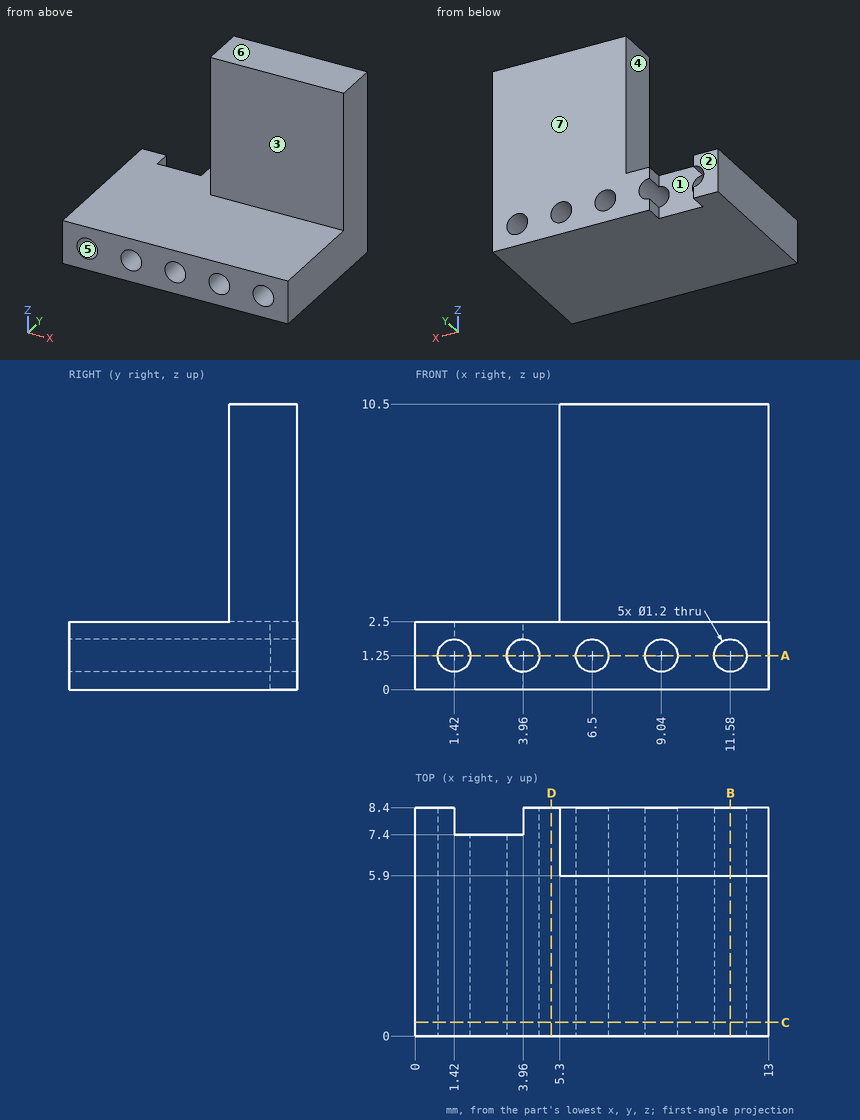
Input: dimensioned drawing with shaded views. Units: mm. Origin: part minimum x, y, z. A direction names the side the tool comes from. Give positions to 0.01 mm unless a question says otherwise; leave off trailing zeros. Loops run counter-clockwise (first coordinate to the right, second up) from the corner with the lowest first, then second, coordinate; pieces in that order, holes last. Notation, with made-up numbers: (6, 77) -> (62, 77) arc R18 ccw to (62, 91) -> close; hole circle Ø7 at (52.25, 7). An arc over 180 degrees is marked (long way). Use a Markdown table: item, result. Add a question column.
1) Section query B-B, the plane x = 11.58. Return the cut outline in (y, z), then the cut area to 3 significant figures.
2) Section query A-A, the plane z = 1.25. Return the cut outline in (x, y).
3) Reachability of the marked faces 1, 2, 3 and 4 from +Z, -Z, +X, -X, +Y, -Y: full face, straight path, thin tool, end or side. Return the list, or none.
4) First-contact query: pin 1 (0.8 mm diameter, centred on y = 7, z = 6, fed in from -X); pin 2 (3 mm diameter, centred on x = 6, z = 5.5, fed in from -Y); pin 3 (0.8 mm diameter, centred on x = 2.5, z = 1.5, fed in from +Y). Flat tips, straight axial feed; report the tip coordinate or a pass-through.
5) Section query C-C, the plane y = 0.5. Return the cut outline in (x, z).
6) Pull-direction query (Z, two-part tool) for the marked faces 5, 6 and 7; classes: +Z half, -Z half, draft (parallel to the pull), parting line (faces both ways), or undercut.
7) Line query: line 1 along X through (y, z) = (8.25, 1.25); line 2 along X through (y, z) = (4.75, 1.25); line 3 along Z through (x, y) = (4, 1.75). Output: solid intervals per line, ascending. Write a range as [from, to].
8) Section query D-D, the plane x = 5. Return the cut outline in (y, z).
Numbers:
| question | item | result |
|---|---|---|
| 1 | outline | (0, 0) -> (8.4, 0) -> (8.4, 0.65) -> (0, 0.65) -> close; (0, 1.85) -> (8.4, 1.85) -> (8.4, 10.5) -> (5.9, 10.5) -> (5.9, 2.5) -> (0, 2.5) -> close |
| 1 | area | 30.9 mm2 |
| 2 | outline | (0, 0) -> (0.82, 0) -> (0.82, 8.4) -> (0, 8.4) -> close; (2.02, 0) -> (3.36, 0) -> (3.36, 7.4) -> (2.02, 7.4) -> close; (4.56, 0) -> (5.9, 0) -> (5.9, 8.4) -> (4.56, 8.4) -> close; (7.1, 0) -> (8.44, 0) -> (8.44, 8.4) -> (7.1, 8.4) -> close; (9.64, 0) -> (10.98, 0) -> (10.98, 8.4) -> (9.64, 8.4) -> close; (12.18, 0) -> (13, 0) -> (13, 8.4) -> (12.18, 8.4) -> close |
| 3 | face 1 | +Z, -Z, +Y |
| 3 | face 2 | +Z, -Z, +X, -X, +Y |
| 3 | face 3 | +Z, +X, -X, -Y |
| 3 | face 4 | +Z, -X, +Y, -Y |
| 4 | pin 1 | stops at x = 5.3 |
| 4 | pin 2 | stops at y = 5.9 |
| 4 | pin 3 | stops at y = 7.4 |
| 5 | outline | (0, 0) -> (13, 0) -> (13, 2.5) -> (0, 2.5) -> close; hole circle Ø1.2 at (1.42, 1.25); hole circle Ø1.2 at (3.96, 1.25); hole circle Ø1.2 at (6.5, 1.25); hole circle Ø1.2 at (9.04, 1.25); hole circle Ø1.2 at (11.58, 1.25) |
| 6 | face 5 | undercut |
| 6 | face 6 | +Z half |
| 6 | face 7 | draft |
| 7 | line 1 | x = [0, 0.82], [4.56, 5.9], [7.1, 8.44], [9.64, 10.98], [12.18, 13] |
| 7 | line 2 | x = [0, 0.82], [2.02, 3.36], [4.56, 5.9], [7.1, 8.44], [9.64, 10.98], [12.18, 13] |
| 7 | line 3 | z = [0, 0.65], [1.85, 2.5] |
| 8 | outline | (0, 0) -> (8.4, 0) -> (8.4, 2.5) -> (0, 2.5) -> close |
